Verification items for the finished model (mm, model axes). Face numbers are marked on the shaded views. A direction names the side the tool comes from. Give positions to 0.01 mm unless a question says otherwise; leave off trailing zeros. Order: outer loops, then holes, each group sorted by start corner. A loop starts at its lowest first (then second) coordinate and runs counter-clockwise, first axis right, second up.
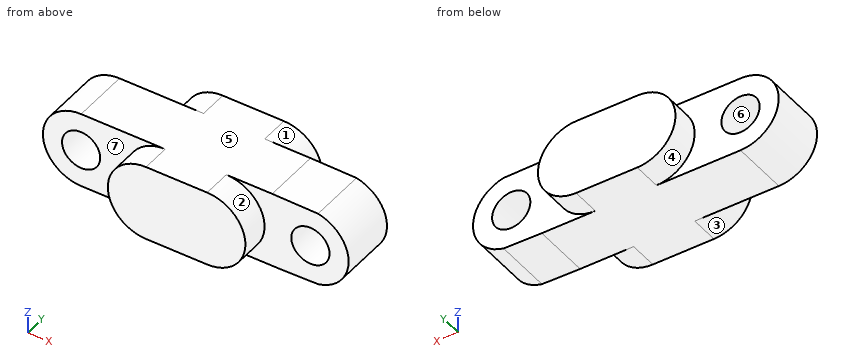
from build123d import *

# Parameters (mm, degrees)
F0_R          = 0.5
F1_DEPTH      = 1.5
F2_DEPTH      = 0.75
F2_DEPTH_BACK = 2.25


# Not quite as in the source:
# - a feature names something its author has since deleted; it is built from what else it names


with BuildPart() as f1:
    # F0 (on Front) → F1 (new body)
    with BuildSketch(Plane.XZ):
        with BuildLine():
            ThreePointArc((-2.4, -2.24940907), (-1.4, -1.24940907), (-2.4, -0.24940907))
            Line((-2.4, -0.24940907), (-4, -0.24940907))
            ThreePointArc((-4, -0.24940907), (-5, -1.24940907), (-4, -2.24940907))
            Line((-4, -2.24940907), (-2.4, -2.24940907))
        make_face()
        with BuildLine():
            Line((0, -0.2696131729), (-1.2, -0.24940907))
            Line((-1.2, -0.24940907), (-2.4, -0.24940907))
            ThreePointArc((-2.4, -0.24940907), (-1.4, -1.24940907), (-2.4, -2.24940907))
            Line((-2.4, -2.24940907), (-1, -2.24940907))
            Line((-1, -2.24940907), (0, -2.2292049671))
            ThreePointArc((0, -2.2292049671), (0.8, -1.24940907), (0, -0.2696131729))
        make_face()
        with Locations((-0.2, -1.24940907)):
            Circle(F0_R, mode=Mode.SUBTRACT)
        with BuildLine():
            ThreePointArc((-4, -2.24940907), (-5, -1.24940907), (-4, -0.24940907))
            Line((-4, -0.24940907), (-6.2, -0.24940907))
            ThreePointArc((-6.2, -0.24940907), (-7.2, -1.24940907), (-6.2, -2.24940907))
            Line((-6.2, -2.24940907), (-4, -2.24940907))
        make_face()
        with Locations((-6.2, -1.24940907)):
            Circle(F0_R, mode=Mode.SUBTRACT)
    extrude(amount=F1_DEPTH)

    # F0 (on Front) → F2 (join, two sides)
    with BuildSketch(Plane.XZ) as f2_sk:
        with BuildLine():
            ThreePointArc((-2.4, -2.24940907), (-1.4, -1.24940907), (-2.4, -0.24940907))
            Line((-2.4, -0.24940907), (-4, -0.24940907))
            ThreePointArc((-4, -0.24940907), (-5, -1.24940907), (-4, -2.24940907))
            Line((-4, -2.24940907), (-2.4, -2.24940907))
        make_face()
    extrude(amount=-F2_DEPTH)
    extrude(f2_sk.sketch, amount=F2_DEPTH_BACK)


solid = f1.part
(1) Scan lines: line 1 (X direction, y = -1.1, z = -1.45); line 2 (X direction, y = -0.9, z = -0.95); line 3 (Y direction, x = -1.5, z = -1.75). Record each from-to range of solid material in increasing order.
Solved:
line 1: x = -7.18 to -6.66, -5.74 to -0.66, 0.26 to 0.78
line 2: x = -7.15 to -6.6, -5.8 to -0.6, 0.2 to 0.75
line 3: y = -1.5 to 0
(2) Release check for a two-part mould opening along Z. For the marked faces 5, 6 and 7 record: pulls with the +Z half, pulls with the -Z half, needs draft (parallel to the pull), parting line crosses it, or undercut.
Solved:
face 5: pulls with the +Z half
face 6: undercut
face 7: needs draft
(3) Section check C-C, the plane z = -1.95. Enter the section's corners in (x, y), then the cut area to 3 significant figures.
Solved:
outline: (-6.91, -1.5) - (-4.71, -1.5) - (-4.71, -2.25) - (-1.69, -2.25) - (-1.69, -1.5) - (0.51, -1.5) - (0.51, 0) - (-1.69, 0) - (-1.69, 0.75) - (-4.71, 0.75) - (-4.71, 0) - (-6.91, 0) - close
area: 15.7 mm2
(4) Section check D-D, the plane z = -1.5. Enter the section's corners in (x, y).
Solved:
outline: (-7.17, -1.5) - (-6.63, -1.5) - (-6.63, 0) - (-7.17, 0) - close; (-5.77, -1.5) - (-4.97, -1.5) - (-4.97, -2.25) - (-1.43, -2.25) - (-1.43, -1.5) - (-0.63, -1.5) - (-0.63, 0) - (-1.43, 0) - (-1.43, 0.75) - (-4.97, 0.75) - (-4.97, 0) - (-5.77, 0) - close; (0.23, -1.5) - (0.77, -1.5) - (0.77, 0) - (0.23, 0) - close
(5) Set-up check for the marked faces 1, 2, 3 and 4: record each of +Z, -Z, +X, -X, +Y, -Y from which the full face is reachable in a straight line by a thin tool's end or side.
Solved:
face 1: +X, +Y
face 2: +X, -Y
face 3: -X, -Y
face 4: -X, +Y
(6) Section check A-A, the plane x = -6. Enter the section's corners in (y, z).
Solved:
outline: (-1.5, -2.25) - (0, -2.25) - (0, -1.71) - (-1.5, -1.71) - close; (-1.5, -0.79) - (0, -0.79) - (0, -0.25) - (-1.5, -0.25) - close
(7) Section check B-B, the plane y = -1.1. Enter the section's corners in (x, z), then the cut area to 3 significant figures.
Solved:
outline: (-6.2, -2.25) - (-1, -2.25) - (0, -2.23) arc R1 ccw to (0, -0.27) - (-1.2, -0.25) - (-6.2, -0.25) arc R1 ccw to start; hole circle Ø1 at (-6.2, -1.25); hole circle Ø1 at (-0.2, -1.25)
area: 13.6 mm2
(8) Go/stop test with a flat-tipped pin: pin 1 (0.6 mm diameter, centred on x = -6, z = -1, fed in from -Y). Record where the tip stops, or that it passes through.
Solved:
pin 1: stops at y = -1.5
